from build123d import *
from build123d.topology import SkipClean

# Parameters (mm, degrees)
RESSALTO_EXTRUS_O1_START = 0.52
RESSALTO_EXTRUS_O1_DEPTH = 0.52


with BuildPart() as part:
    # Esboço1 → Revolução1 (revolve)
    with BuildSketch(Plane.XY, mode=Mode.PRIVATE) as revolu_o1_sk:
        Polygon((0.38, 2.7), (15.8, 2.7), (16, 2.646410162), (16, 2.4), (4.100420175, 2.3), (4.100420175, 1.8), (3.67, 1.8), (3.67, 2.3), (0, 2.3), (0, 3.15), (0.38, 3.15), align=None)
    revolve(revolu_o1_sk.sketch.rotate(Axis((0, 0, 0), (1, 0, 0)), 90), axis=Axis((0, 0, 0), (1, 0, 0)))

    # Esboço3 → Ressalto-extrusão1 (add)
    with SkipClean():  # the faces are left unmerged after this step: merging them gives an invalid solid
        with BuildSketch(Plane(origin=(0.38, 0, 0), x_dir=(0, 0, -1), z_dir=(1, 0, 0)).offset(RESSALTO_EXTRUS_O1_START)):
            with BuildLine():
                Line((-3.110064308, 0.5), (-2.653299832, 0.5))
                ThreePointArc((-2.653299832, 0.5), (-2.7, 0), (-2.653299832, -0.5))
                Line((-2.653299832, -0.5), (-3.110064308, -0.5))
                ThreePointArc((-3.110064308, -0.5), (-3.15, 0), (-3.110064308, 0.5))
            make_face()
            with BuildLine():
                Line((2.653299832, -0.5), (3.110064308, -0.5))
                ThreePointArc((3.110064308, -0.5), (3.15, 0), (3.110064308, 0.5))
                Line((3.110064308, 0.5), (2.653299832, 0.5))
                ThreePointArc((2.653299832, 0.5), (2.7, 0), (2.653299832, -0.5))
            make_face()
        extrude(amount=-RESSALTO_EXTRUS_O1_DEPTH)


solid = part.part
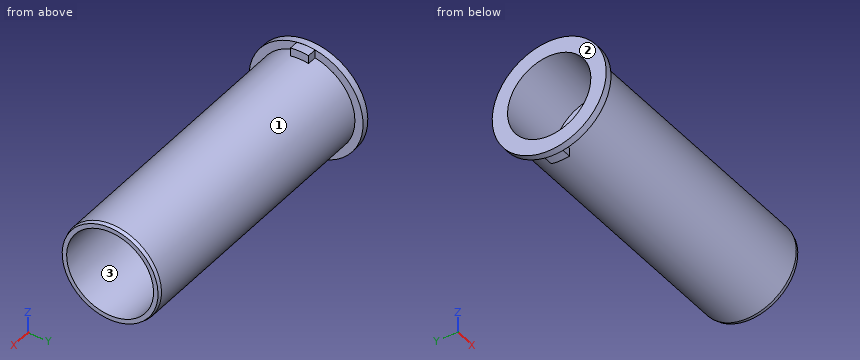
CAD build for the part. Positions are in the model's coordinates, mm. Face numbers are marked on the shaded views. Coordinates: 2 decimals unless noted, no trailing zeros. Order: outer loops, then holes, each group sorted by start corner. A loop starts at its lowest first (then second) coordinate and runs counter-clockwise, first axis right, second up.
Item 1: Band-saw the part on A-A on x = 2.5. List the corners of the cut face in (y, z).
Check sheet entries:
outline: circle Ø5.4 at (0, 0); hole circle Ø4.6 at (0, 0)
Item 2: Band-saw the part on B-B on x = 10.5. List the corners of the cut face in (y, z), plus the area to 3 significant figures.
Check sheet entries:
outline: circle Ø5.4 at (0, 0); hole circle Ø4.71 at (0, 0)
area: 5.50 mm2
Item 3: Pin check, flat tips, straight feed: pin 1 Ø1 at (x, z) = (6.5, 1) entering from +Y; pin 2 Ø2 at (y, z) = (-0.5, -1) entering from -X; pin 3 Ø0.5 at (x, z) = (1, -3) entering from +Y. Stop position of each tip, or through.
Check sheet entries:
pin 1: stops at y = 2.65
pin 2: stops at x = 3.67
pin 3: stops at y = 0.5
Item 4: Drill centre lines: L1, parallel to Y at x = 2.5, z = 0; L2, parallel to Y at x = 3.85, z = 0; L3, parallel to X at y = 1.25, z = 1.75. Where is each one in solid material? Low to high.
Check sheet entries:
L1: y = -2.7 to -2.3, 2.3 to 2.7
L2: y = -2.7 to -1.8, 1.8 to 2.7
L3: x = 3.67 to 4.1
Item 5: Two-plate mould, pull along Z, no slides. Class the marked faces 1, 2 and 3: +Z half, -Z half, draft (parallel to the pull), parting line (faces both ways), or undercut.
Check sheet entries:
face 1: parting line
face 2: draft
face 3: undercut
